Verification items for the finished model (mm, model axes). A direction names the side the tool comes from. Give positions to 0.01 mm unless a question says otherwise; leave off trailing zeros. Order: outer loops, then holes, each group sorted by start corner. A loop starts at its lowest first (then second) coordinate and runs counter-clockwise, first axis right, second up. Notation, with made-up numbers: (54.5, 39) - (102.5, 39) arc R23 cw to (102.5, 68) - close; hole circle Ø1 at (53, -30.75). An arc over 180 degrees is marked (long way). Answer as a JSON object with one key per item and string values. Group by question number.
(1) Thickness scan on line 1 (Y direction, x = 0, z = 10.5); line 2 (Z direction, x = -2.25, y = 1); line 3 (X direction, y = -0.45, z = 7). Record the ranges inside material, lowest first.
(2) Depth check by flat-ended pin: pin 1 Ø1.5 at (x, y) = (-2, 1.5) entering from -Z; pin 2 Ø1.2 at (x, y) = (-0.5, 0) entering from +Z. Enter the tip coordinate at first touch or a pass-through.
(3) Section check A-A (z = 5.75). Record the boundary of the cut face in (x, y).
(4) Access from +Z, -Z, +X, -X, +Y, -Y to the whole of each face (thin tool, end or side, straight path). Record for faces 1 (the face through (0, 0, 6)), 2 (the face through (1.31, -2.29, 11.86)), 3 (the face through (-1.25, -0.05, -1.38)).
(5) Mould release check, pull along X, two halves, no side actions. Record for faces 4 (the face through (-1.323, -2.279, 11.865)), 5 (the face through (-0.27, -1.22, 8.94)), 6 (the face through (1, 1, 0)): +X half, -X half, draft (parallel to the pull), parting line (faces both ways), or undercut.
```python
from build123d import *

# Parameters (mm, degrees)
BOSS_EXTRU_1_DEPTH      = 12
ESQUISSE3_R             = 1.25
ENL_V_MAT_EXTRU_1_DEPTH = 6
CHANFREIN1_SIZE         = 0.2
ESQUISSE4_R             = 1.25
BOSS_EXTRU_2_DEPTH      = 3
CHANFREIN2_SIZE         = 0.2


with BuildPart() as part:
    # Esquisse1 → Boss.-Extru.1 (new body)
    with BuildSketch(Plane.XY):
        Polygon((2.886751346, 0), (1.443375673, 2.5), (-1.443375673, 2.5), (-2.886751346, 0), (-1.443375673, -2.5), (1.443375673, -2.5), align=None)
    extrude(amount=BOSS_EXTRU_1_DEPTH)

    # Esquisse2 → Enlèvement de matière-Révolution1 (revolve, cut)
    with BuildSketch(Plane(origin=(0, 0, 0), x_dir=(1, 0, 0), z_dir=(0, 1, 0))):
        Polygon((-1.5, 1), (-3, -0.5), (-3, 1), align=None)
        Polygon((-3, -11.5), (-1.5, -13), (-3, -13), align=None)
    revolve(axis=Axis((0, 0, 0), (0, 0, 1)), mode=Mode.SUBTRACT)

    # Esquisse3 → Enlèv. mat.-Extru.1 (cut)
    with BuildSketch(Plane.XY.offset(12)):
        Circle(ESQUISSE3_R)
    extrude(amount=-ENL_V_MAT_EXTRU_1_DEPTH, mode=Mode.SUBTRACT)

    # Chanfrein1
    chanfrein1_edges = [part.edges().sort_by_distance(p)[0] for p in [
        (-1.25, 0, 12),
    ]]
    chamfer(chanfrein1_edges, length=CHANFREIN1_SIZE)

    # Esquisse4 → Boss.-Extru.2 (add)
    with BuildSketch(Plane(origin=(0, 0, 0), x_dir=(-1, 0, 0), z_dir=(0, 0, -1))):
        with Locations(Location((0, 0, 0), (0, 0, 180))):
            Circle(ESQUISSE4_R)
    extrude(amount=BOSS_EXTRU_2_DEPTH)

    # Chanfrein2
    chanfrein2_edges = [part.edges().sort_by_distance(p)[0] for p in [
        (-1.25, 0, -3),
    ]]
    chamfer(chanfrein2_edges, length=CHANFREIN2_SIZE)


solid = part.part
```
Solutions:
{
 "1": {"line 1": "y = -2.5 to -1.25, 1.25 to 2.5", "line 2": "z = 0 to 12", "line 3": "x = -2.63 to -1.17, 1.17 to 2.63"},
 "2": {"pin 1": "stops at z = 0", "pin 2": "stops at z = 6"},
 "3": {"outline": "(-2.89, 0) - (-1.44, -2.5) - (1.44, -2.5) - (2.89, 0) - (1.44, 2.5) - (-1.44, 2.5) - close"},
 "4": {"face 1": "+Z", "face 2": "+Z, +X, -Y", "face 3": "-Z"},
 "5": {"face 4": "-X half", "face 5": "undercut", "face 6": "draft"}
}
